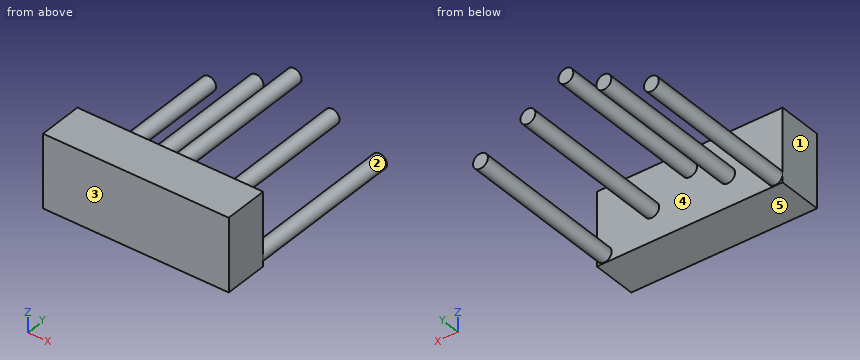
```python
from build123d import *

# Parameters (mm, degrees)
SKETCH1_W           = 79.502
SKETCH1_H           = 31.242
BOSS_EXTRUDE1_DEPTH = 19.05
SKETCH2_R           = 3.175
BOSS_EXTRUDE2_DEPTH = 68.58


with BuildPart() as part:
    # Sketch1 → Boss-Extrude1 (new body)
    with BuildSketch(Plane(origin=(0, 0, 0), x_dir=(1, 0, 0), z_dir=(0, 1, 0))):
        Rectangle(SKETCH1_W, SKETCH1_H)
    extrude(amount=BOSS_EXTRUDE1_DEPTH)

    # Sketch2 → Boss-Extrude2 (add)
    with BuildSketch(Plane(origin=(0, 19.05, 0), x_dir=(1, 0, 0), z_dir=(0, 1, 0))):
        with Locations(Location((-36.576, 12.192, 0), (0, 0, 180))):
            Circle(SKETCH2_R)
        with Locations(Location((-16.256, 2.515131479, 0), (0, 0, 270))):
            Circle(SKETCH2_R)
        with Locations(Location((0, -7.263868521, 0), (0, 0, 270))):
            Circle(SKETCH2_R)
        with Locations(Location((16.256, 2.515131479, 0), (0, 0, 270))):
            Circle(SKETCH2_R)
        with Locations((36.576, 12.192)):
            Circle(SKETCH2_R)
    extrude(amount=BOSS_EXTRUDE2_DEPTH)


solid = part.part
```
Design review of the part built by this model. Coordinates are the model's own, in mm. Face numbers are marked on the shaded views. A direction names the side the tool comes from. Give positions to 0.01 mm unless a question says otherwise; leave off trailing zeros. Write each loop counter-clockwise with the first axis right and the second up, starting at its lowest first coordinate (ties: lowest second). Pieces come first, ordered by that corner, then holes. Notation, with made-up numbers: (-23.5, 68) - (-2.5, 68) arc R25 ccw to (-2.5, 105) - close; hole circle Ø1 at (-37.75, 82.5). An arc over 180 degrees is marked (long way). Return JSON: item names as keys, results as strings. Group by question number.
(1) We need section D-D, the plane x = 30. Give the boundary of the cut face in (y, z), then the cut area to 3 significant figures.
(2) Machinability: for the marked faces 4 and 5, which of the approach directions +Z, -Z, +X, -X, +Y, -Y give a long, thin tool a straight path to every point of the face, cutting with its end or side? Answer none if there is none.
(3) Insertion check: pin 1 (6 mm diameter, centred on x = -17.5, y = 78, fed in from -Z); pin 2 (3 mm diameter, centred on x = 11.5, y = 56.5, fed in from -Z); pin 3 (4 mm diameter, centred on y = 75, z = -8, fed in from -X); pin 4 (5 mm diameter, centred on x = 19, y = 51.5, fed in from +Z). Each pin has a flat end and moves straight along its axis. Give the tip position at first contact, or say it passes through.
(4) We need section C-C, the plane y = 67.5. Give the boundary of the cut face in (x, z) (3 decimals).
(5) Mouldability with a two-part tool opening along X and no side actions: class the marked faces 1, 2 and 3 as +X half, -X half, draft (parallel to the pull), parting line (faces both ways), or undercut.
(6) We need section B-B, the plane z = 13. Give the boundary of the cut face in (x, y), then the cut area to 3 significant figures.
(7) We need section A-A, the plane x = 0. Give the boundary of the cut face in (y, z).
(8) To check wall thickness, follow probe 1 along Y at (x, z) = (-32.5, -3.5); probe 2 along X at (y, z) = (50.5, -13.5); probe 3 along X at (y, z) = (77.5, -1). State the ranges of each line that lie inside material, in increasing order.
Reported:
{
 "1": {"outline": "(0, -15.62) - (19.05, -15.62) - (19.05, 15.62) - (0, 15.62) - close", "area": "595 mm2"},
 "2": {"face 4": "+Y", "face 5": "-Z, +X, -X, +Y, -Y"},
 "3": {"pin 1": "stops at z = -5.69", "pin 2": "passes through", "pin 3": "stops at x = -38.87", "pin 4": "stops at z = 0.65"},
 "4": {"outline": "circle Ø6.35 at (-36.576, -12.192); circle Ø6.35 at (-16.256, -2.515); circle Ø6.35 at (0, 7.264); circle Ø6.35 at (16.256, -2.515); circle Ø6.35 at (36.576, -12.192)"},
 "5": {"face 1": "-X half", "face 2": "undercut", "face 3": "draft"},
 "6": {"outline": "(-39.75, 0) - (39.75, 0) - (39.75, 19.05) - (-39.75, 19.05) - close", "area": "1,510 mm2"},
 "7": {"outline": "(0, -15.62) - (19.05, -15.62) - (19.05, 4.09) - (87.63, 4.09) - (87.63, 10.44) - (19.05, 10.44) - (19.05, 15.62) - (0, 15.62) - close"},
 "8": {"probe 1": "y = 0 to 19.05", "probe 2": "x = -39.47 to -33.68, 33.68 to 39.47", "probe 3": "x = -19.05 to -13.47, 13.47 to 19.05"}
}
